```python
from build123d import *

# Parameters (mm, degrees)
SKETCH1_R           = 12.7
BOSS_EXTRUDE1_DEPTH = 2.5
BOSS_EXTRUDE2_DEPTH = 2.5
CIRPATTERN1_COUNT   = 22
SKETCH3_R           = 0.75
CUT_EXTRUDE1_DEPTH  = 5


with BuildPart() as part:
    # Sketch1 → Boss-Extrude1 (new body)
    with BuildSketch(Plane(origin=(0, 0, 0), x_dir=(1, 0, 0), z_dir=(0, 1, 0))):
        with Locations(Location((0, 0, 0), (0, 0, 270))):
            Circle(SKETCH1_R)
    extrude(amount=BOSS_EXTRUDE1_DEPTH)

    # Sketch2 → Boss-Extrude2 (add)
    with BuildSketch(Plane(origin=(0, 2.5, 0), x_dir=(1, 0, 0), z_dir=(0, 1, 0))):
        Polygon((-1.324709139, 12.192), (1.324709139, 12.192), (0.508, 15.24), (-0.508, 15.24), align=None)
    boss_extrude2 = extrude(amount=-BOSS_EXTRUDE2_DEPTH)

    # CirPattern1: Boss-Extrude2 ×22 about axis
    cirpattern1_axis = Axis((0, 0, 0), (0, 1, 0))
    for i in range(1, CIRPATTERN1_COUNT):
        add(boss_extrude2.rotate(cirpattern1_axis, i * 360 / CIRPATTERN1_COUNT))

    # Sketch3 → Cut-Extrude1 (cut)
    with BuildSketch(Plane(origin=(0, 2.5, 0), x_dir=(1, 0, 0), z_dir=(0, 1, 0))):
        with Locations(Location((0, 0, 0), (0, 0, 270))):
            Circle(SKETCH3_R)
    extrude(amount=-CUT_EXTRUDE1_DEPTH, mode=Mode.SUBTRACT)


solid = part.part
```
Could you check a few things on this model? Use its own coordinates, in mm. A direction names the side the tool comes from. Coordinates: 2 decimals unless noted, no trailing zeros. Write each loop counter-clockwise with the first axis right and the second up, starting at its lowest first coordinate (ties: lowest second). Pieces come first, ordered by that corner, then holes. Notation, with made-up numbers: (40, -11.5) -> (50, -11.5) arc R23 ccw to (50, 2.5) -> close; hole circle Ø11 at (-34, -7). An arc over 180 degrees is marked (long way). Write item = value, one per line. Start each with the question number.
(1) Which directions (+Z, -Z, +X, -X, +Y, -Y) give clear straight access to the entire face, cutting with the end or side of a thin tool? Please do faces 1 (the face through (13.939, 1.268, 1.144)), 2 (the face through (8.323, 1.232, -9.592)), 3 (the face through (-13.052, 1.268, -5.025)), 4 (the face through (-6.803, 1.268, -12.178)), 5 (the face through (9.96, 1.27, 9.77)).
(2) I want a section at C-C (z = 8). Please give me the cut outline in (x, y), plus the area to 4 significant figures.
(3) I want a section at B-B (z = 0). Please give me the cut outline in (x, y).
(4) Will these pins go through, and if not, where does the flat tip stop? pin 1 (1 mm diameter, centred on y = 1.5, z = 6.5, fed in from -X); pin 2 (1.5 mm diameter, centred on y = 1, z = 11.5, fed in from -X); pin 3 (1.5 mm diameter, centred on x = -9.5, y = 1, fed in from +Z).
(5) We'd pull the mould along X, two halves only. Please class faces 6 (the face through (-15.086, 1.268, 2.162)), 7 (the face through (-9.993, 1.268, 9.785)), 8 (the face through (13.904, 1.268, -1.129)): released by +X, released by -X, zero draft, split by the parting line, or undercut.
(6) I want a section at A-A (x = 0). Please give me the cut outline in (y, z), plus the area to 4 significant figures.
(7) I need wall thicknesses on line 1 (Z direction, x = 11.5, y = 2.2); line 2 (Z direction, x = 12.5, y = 0.95); line 3 (Z direction, x = 14.5, y = 0.9). Which ranges of each line are inside material? Lowest first, please. Write a range as [from, to].
Result set:
q1.face_1 = +X, +Y, -Y
q1.face_2 = +Y, -Y
q1.face_3 = -X, +Y, -Y
q1.face_4 = -Z, +Y, -Y
q1.face_5 = +Z, +Y, -Y
q2.outline = (-10.77, 0) -> (10.77, 0) -> (10.77, 2.5) -> (-10.77, 2.5) -> close
q2.area = 53.85 mm2
q3.outline = (-12.7, 0) -> (-0.75, 0) -> (-0.75, 2.5) -> (-12.7, 2.5) -> close; (0.75, 0) -> (12.7, 0) -> (12.7, 2.5) -> (0.75, 2.5) -> close
q4.pin_1 = -14.01
q4.pin_2 = -8.57
q4.pin_3 = 9.91
q5.face_6 = released by -X
q5.face_7 = undercut
q5.face_8 = released by +X
q6.outline = (0, -15.24) -> (2.5, -15.24) -> (2.5, -0.75) -> (0, -0.75) -> close; (0, 0.75) -> (2.5, 0.75) -> (2.5, 15.24) -> (0, 15.24) -> close
q6.area = 72.45 mm2
q7.line_1 = [-10, -9.08], [-6.43, 6.43], [9.08, 10]
q7.line_2 = [-6.6, -4.57], [-2.97, 2.97], [4.57, 6.6]
q7.line_3 = [-2.73, -1.38], [1.38, 2.73]
